Source: CAD feature listing. Evaluate the final solid. Frame: model axes, mm. A direction names the side the tool comes from. Round coordinates to 2 decimals unless told otherwise and drop trailing zeros. Loops run counter-clockwise (first coordinate to the right, second up) from the corner with the lowest first, then second, coordinate; pieces in that order, holes last. Notation, with made-up numbers: (20.5, 88) -> (53.5, 88) arc R17 cw to (53.5, 121) -> close; hole circle Ø11 at (22.25, 70.25). An arc over 180 degrees is marked (long way). Put each result on its own line as item: value. Start each with the question number.
1. Draft query along Y for faces 3 (the flat face through (50, 1, 17)), 4 (the flat face through (-3.235, 17, 18)), 5 (the flat face through (1, -50, 17)). Return one class per face: pulls with the +Y half, pulls with the -Y half, needs draft (parallel to the pull), parting line crosses it, or undercut.
2. Cut plane A-A (x = 0). Return the cut outline in (y, z).
3. Set-up query: faces 1 (the flat face through (0, 18.647, 18)), 2 (the flat face through (-50, -1, 17)). Return all of +Z, -Z, +X, -X, +Y, -Y with unobstructed straight access to the full face (end or side cutting, diameter ignored); none if empty.
4. Cut plane B-B (y = 0). Return the cut outline in (x, z).
5. Cut plane C-C (z = 5). Return the cut outline in (x, y) (3 decimals).
6. Material intervals for L1, parallel to Y at x = 0, z = 26.5; L2, parallel to X at y = 0, z = 18; L3, parallel to X at y = -12, z = 6, sorted ascending.
```python
from build123d import *

# Parameters (mm, degrees)
BOSS_EXTRUDE1_DEPTH = 35
SKETCH2_R           = 15
CUT_EXTRUDE1_DEPTH  = 50


with BuildPart() as part:
    # Sketch1 → Boss-Extrude1 (new body)
    with BuildSketch(Plane.XY):
        Polygon((24.650973025, 50), (50, 50), (50, -50), (-50, -50), (-50, 50), align=None)
    extrude(amount=BOSS_EXTRUDE1_DEPTH)

    # Sketch2 → Cut-Extrude1 (cut)
    with BuildSketch(Plane.XY.offset(35)):
        Circle(SKETCH2_R)
        with BuildLine():
            Line((3.235, 18.647005667), (-3.235, 18.647005667))
            Line((-3.235, 18.647005667), (-3.235, 14.647005667))
            ThreePointArc((-3.235, 14.647005667), (0, 15), (3.235, 14.647005667))
            Line((3.235, 14.647005667), (3.235, 18.647005667))
        make_face()
    extrude(amount=-CUT_EXTRUDE1_DEPTH, mode=Mode.SUBTRACT)


solid = part.part
```
Solution:
1. face 3: needs draft
1. face 4: undercut
1. face 5: pulls with the -Y half
2. outline: (-50, 0) -> (-15, 0) -> (-15, 35) -> (-50, 35) -> close; (18.65, 0) -> (50, 0) -> (50, 35) -> (18.65, 35) -> close
3. face 1: +Z, -Z
3. face 2: +Z, -Z, -X, +Y, -Y
4. outline: (-50, 0) -> (-15, 0) -> (-15, 35) -> (-50, 35) -> close; (15, 0) -> (50, 0) -> (50, 35) -> (15, 35) -> close
5. outline: (-50, -50) -> (50, -50) -> (50, 50) -> (-50, 50) -> close; hole (-3.235, 14.647) arc R15 ccw (long way) to (3.235, 14.647) -> (3.235, 18.647) -> (-3.235, 18.647) -> close
6. L1: y = -50 to -15, 18.65 to 50
6. L2: x = -50 to -15, 15 to 50
6. L3: x = -50 to -9, 9 to 50
